Here's the drawing with two shaded views (mm, measured from the low corner). I have some questions. Round coordinates to 2 decimals unless told otherwise and drop trailing zeros. Write each loop counter-clockwise with the first axis right and the second up, starting at its lowest first coordinate (ties: lowest second). Pieces come first, ordered by that corner, then holes. Notation, with made-up numbers: (25.25, 80.5) -> (65.25, 80.5) arc R17 cw to (65.25, 113.5) -> close; hole circle Ø9 at (19.25, 47.5). An arc over 180 degrees is marked (long way). Use CSV: the item, a comma, the result in double quotes.
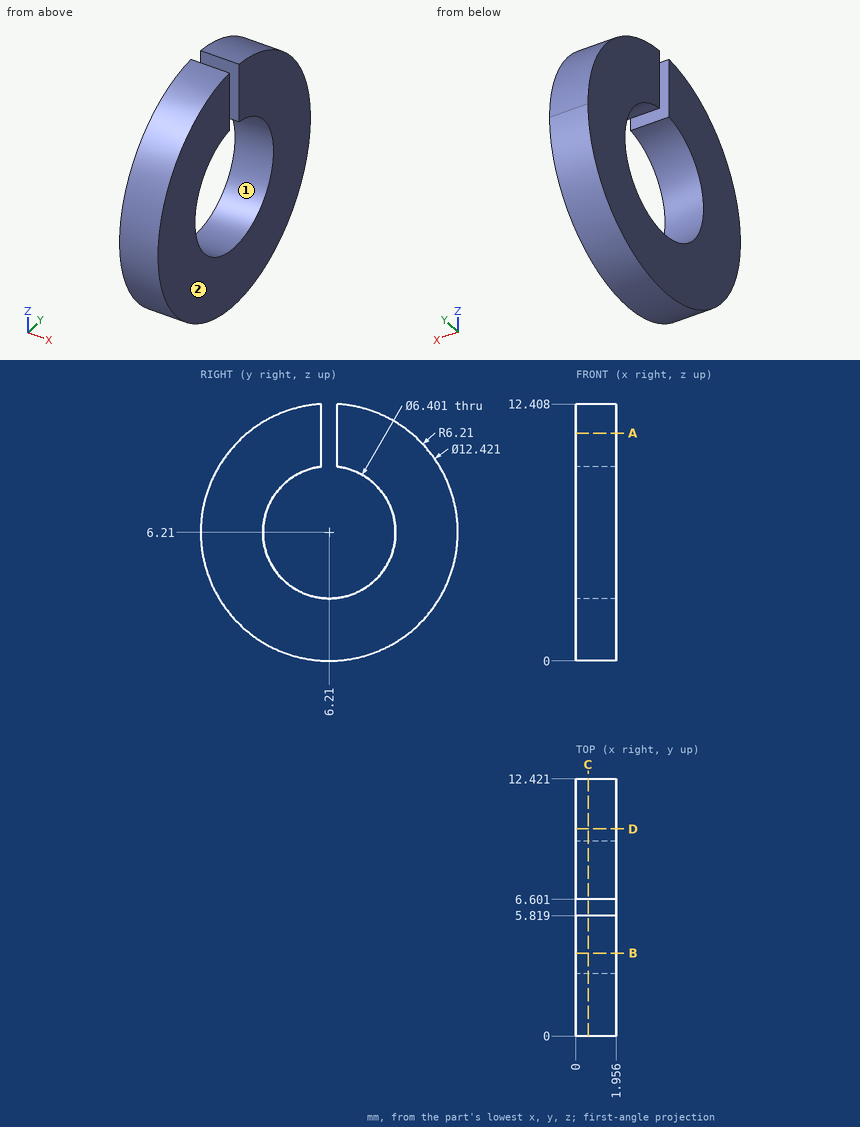
Q1. Suppose I cut it at C-C (x = 0.6). Write out the boundary of the cut face in (y, z).
Resolved:
outline,"(5.82, 9.39) -> (5.82, 12.41) arc R6.21 ccw (long way) to (6.6, 12.41) -> (6.6, 9.39) arc R3.2 cw (long way) to start"
Q2. Suppose I cut it at D-D (y = 10). Write out the boundary of the cut face in (x, z) (1 decimal).
Resolved:
outline,"(0, 1.3) -> (2, 1.3) -> (2, 11.1) -> (0, 11.1) -> close"
Q3. Please list where these lines run through material, in increasing order: probe 1 along Z at (x, y) = (0.85, 5.5); probe 2 along Z at (x, y) = (0.35, 5.75); probe 3 along Y at (x, z) = (1, 11.5) (1 decimal).
Resolved:
probe 1,"z = 0.04 to 3.09, 9.33 to 12.38"
probe 2,"z = 0.02 to 3.04, 9.38 to 12.4"
probe 3,"y = 3 to 5.8, 6.6 to 9.5"
Q4. Suppose I cut it at A-A (z = 11). Write out the boundary of the cut face in (x, y) (1 decimal).
Resolved:
outline,"(0, 2.3) -> (2, 2.3) -> (2, 5.8) -> (0, 5.8) -> close; (0, 6.6) -> (2, 6.6) -> (2, 10.2) -> (0, 10.2) -> close"
Q5. Suppose I cut it at B-B (y = 4). Write out the boundary of the cut face in (x, z) (1 decimal).
Resolved:
outline,"(0, 0.4) -> (2, 0.4) -> (2, 3.9) -> (0, 3.9) -> close; (0, 8.5) -> (2, 8.5) -> (2, 12) -> (0, 12) -> close"
Q6. If we mould it in two halves opening along Z, with no side actions, what happens to the marked faces 1 and 2? For each: released by +Z, released by -Z, zero draft, split by the parting line, or undercut.
Resolved:
face 1,"undercut"
face 2,"zero draft"
Q7. Will these pins go through, and if not, where does the flat tip stop? P1, Ø0.6, axis at x = 1.5, z = 11, coming from the +Y side; P2, Ø1, axis at x = 1.5, z = 9.5, coming from the -Y side; P3, Ø1, axis at x = 1, z = 11, coming from the -Y side.
Resolved:
P1,"stops at y = 10.5"
P2,"stops at y = 0.66"
P3,"stops at y = 1.72"
